```python
from build123d import *

# Parameters (mm, degrees)
F0_W     = 38.1
F0_H     = 114.3
F1_DEPTH = 38.1


with BuildPart() as f1:
    # F0 (on Front) → F1 (new body)
    with BuildSketch(Plane.XZ):
        Polygon((-457.014564, 38.1), (-457.014564, 0), (990.785436, 0), (990.785436, 38.1), (952.685436, 38.1), (-418.914564, 38.1), align=None)
        Polygon((952.685436, 38.1), (990.785436, 38.1), (990.785436, 723.9), (952.685436, 723.9), (952.685436, 676.546395), align=None)
        Polygon((-418.914564, 876.3), (-418.914564, 838.2), (-164.914564, 838.2), (-126.814564, 838.2), (660.585436, 838.2), (698.685436, 838.2), (952.685436, 838.2), (952.685436, 876.3), align=None)
        Polygon((-457.014564, 1028.7), (-457.014564, 723.9), (-418.914564, 723.9), (-418.914564, 838.2), (-418.914564, 876.3), (-418.914564, 1028.7), align=None)
        Polygon((-457.014564, 723.9), (-457.014564, 38.1), (-418.914564, 38.1), (-418.914564, 676.546395), (-418.914564, 723.9), align=None)
        Polygon((952.685436, 723.9), (990.785436, 723.9), (990.785436, 1028.7), (952.685436, 1028.7), (952.685436, 876.3), (952.685436, 838.2), align=None)
        with Locations((-145.864564, 781.05)):
            Rectangle(F0_W, F0_H)
        Polygon((-418.914564, 723.9), (-418.914564, 676.546395), (952.685436, 676.546395), (952.685436, 723.9), (698.685436, 723.9), (660.585436, 723.9), (-126.814564, 723.9), (-164.914564, 723.9), align=None)
        with Locations((679.635436, 781.05)):
            Rectangle(F0_W, F0_H)
    extrude(amount=F1_DEPTH)


solid = f1.part
```
Can you work these out from the model? Positions are in its coordinate system, mm. A direction names the side the tool comes from. Coordinates: 2 decimals unless noted, no trailing zeros. Order: outer loops, then holes, each group sorted by start corner. A loop starts at its lowest first (then second) coordinate and runs counter-clockwise, first axis right, second up.
1. I'm going to push a flat-ended pin straight in: pin 1 (19 mm diameter, centred on x = 776.5, y = -25.5, fed in from +Z). Where does the tip first touch, or does it pass through?
2. If we section it at B-B (x = 853): Please give me the cut outline in (y, z), then the cut area to 3 significant figures.
3. If we section it at C-C (y = -21): Please give me the cut outline in (x, z), then the cut area to 3 significant figures.
4. If we section it at D-D (z = 157): Please give me the cut outline in (x, y).
5. I need wall thicknesses on line 1 (Z direction, x = 156, y = -23); line 2 (X direction, y = -16.5, z = 780); line 3 (X direction, y = -28.5, z = 425.5). Which ranges of each line are inside material? Lowest first, please.
6. If we section it at A-A (z = 755): Please give me the cut outline in (x, y), then the cut area to 3 significant figures.
7. For faces 4 (the face through (257, -19, 0)), 5 (the face through (-418.915, -19, 951)), 6 (the face through (276, -19, 38.1)), which set-ups out of +Z, -Z, +X, -X, +Y, -Y let a thin tool reach every point of the face, with its end or its side?
8. Thinking about a two-plate mould opening in X: for faces 1 (the face through (952.685, -19, 362)), 2 (the face through (990.785, -19, 507)), 3 (the face through (972, -19, 1028.7)), which applies, +X half, -X half, draft (parallel to the pull), parting line (faces both ways), or undercut?
Entries:
1. pin 1: stops at z = 876.3
2. outline: (-38.1, 0) - (0, 0) - (0, 38.1) - (-38.1, 38.1) - close; (-38.1, 676.55) - (0, 676.55) - (0, 723.9) - (-38.1, 723.9) - close; (-38.1, 838.2) - (0, 838.2) - (0, 876.3) - (-38.1, 876.3) - close
2. area: 4,710 mm2
3. outline: (-457.01, 0) - (990.79, 0) - (990.79, 1028.7) - (952.69, 1028.7) - (952.69, 876.3) - (-418.91, 876.3) - (-418.91, 1028.7) - (-457.01, 1028.7) - close; hole (-418.91, 38.1) - (952.69, 38.1) - (952.69, 676.55) - (-418.91, 676.55) - close; hole (-418.91, 723.9) - (-164.91, 723.9) - (-164.91, 838.2) - (-418.91, 838.2) - close; hole (-126.81, 723.9) - (660.59, 723.9) - (660.59, 838.2) - (-126.81, 838.2) - close; hole (698.69, 723.9) - (952.69, 723.9) - (952.69, 838.2) - (698.69, 838.2) - close
3. area: 257,000 mm2
4. outline: (-457.01, -38.1) - (-418.91, -38.1) - (-418.91, 0) - (-457.01, 0) - close; (952.69, -38.1) - (990.79, -38.1) - (990.79, 0) - (952.69, 0) - close
5. line 1: z = 0 to 38.1, 676.55 to 723.9, 838.2 to 876.3
5. line 2: x = -457.01 to -418.91, -164.91 to -126.81, 660.59 to 698.69, 952.69 to 990.79
5. line 3: x = -457.01 to -418.91, 952.69 to 990.79
6. outline: (-457.01, -38.1) - (-418.91, -38.1) - (-418.91, 0) - (-457.01, 0) - close; (-164.91, -38.1) - (-126.81, -38.1) - (-126.81, 0) - (-164.91, 0) - close; (660.59, -38.1) - (698.69, -38.1) - (698.69, 0) - (660.59, 0) - close; (952.69, -38.1) - (990.79, -38.1) - (990.79, 0) - (952.69, 0) - close
6. area: 5,810 mm2
7. face 4: -Z, +X, -X, +Y, -Y
7. face 5: +Z, +Y, -Y
7. face 6: +Y, -Y
8. face 1: undercut
8. face 2: +X half
8. face 3: draft
